from build123d import *

# Parameters (mm, degrees)
F0_R     = 29
F1_DEPTH = 135
F4_DEPTH = 10
F5_DEPTH = 10


with BuildPart() as f1:
    # F0 (on Right) → F1 (new body)
    with BuildSketch(Plane.YZ):
        Circle(F0_R)
    extrude(amount=-F1_DEPTH)

    # F2 (on Right) → F3 (revolve)
    with BuildSketch(Plane.YZ):
        with BuildLine():
            ThreePointArc((0, 16), (3.1819805153, 17.3180194847), (4.5, 20.5))
            ThreePointArc((4.5, 20.5), (-3.1819805153, 23.6819805153), (0, 16))
        make_face()
    revolve(axis=Axis((0, -100, 0), (0, -1, 0)))

    # F4 (add): a face of the model
    f4_faces = [f1.faces().sort_by_distance(p)[0] for p in [
        (-135, 0, 0),
    ]]
    extrude(f4_faces, amount=F4_DEPTH)

    # F5 (cut): a face of the model
    f5_faces = [f1.faces().sort_by_distance(p)[0] for p in [
        (0, 0, 0),
    ]]
    extrude(f5_faces, amount=-F5_DEPTH, mode=Mode.SUBTRACT)


solid = f1.part
Check sheet for the modelled part. Datum: model origin and axes. Units: mm. Round coordinates to 2 decimals unless told otherwise and drop trailing zeros. Loops run counter-clockwise (first coordinate to the right, second up) from the corner with the lowest first, then second, coordinate; pieces in that order, holes last. Notation, with made-up numbers: (-32.75, 67) - (26.25, 67) arc R19 ccw to (26.25, 91) - close; hole circle Ø5 at (19.5, 70.5). An arc over 180 degrees is marked (long way). Answer as CSV lines item,"result". Start each with the question number.
Item 1: Section check A-A (x = -6). Record the boundary of the cut face in (y, z), and give its area (3 significant figures).
Item 2: Section check C-C (x = -45.5). Record the boundary of the cut face in (y, z).
Item 3: Section check D-D (y = 18). Record the boundary of the cut face in (x, z).
Item 4: Depth check by flat-ended pin: P1, Ø6, axis at x = -72.5, y = 18.5, coming from the +Z side; P2, Ø12, axis at x = -107, y = 6.5, coming from the +Z side; P3, Ø4, axis at y = 0, z = -9.5, coming from the +X side. Enter the tip coordinate at first touch or a pass-through.
Item 5: Section check B-B (y = -16.5). Record the boundary of the cut face in (x, z).
Item 6: Scan lines: line 1 (X direction, y = 25, z = 13.5); line 2 (Y direction, x = -36, z = 20.5); line 3 (X direction, y = 3.5, z = 13.5). Record each from-to range of solid material in increasing order. Write a range as [from, to].
Report:
1,outline,"circle Ø9 at (0, -20.5); circle Ø9 at (0, 20.5)"
1,area,"127 mm2"
2,outline,"circle Ø58 at (0, 0)"
3,outline,"(-145, -22.74) - (-10, -22.74) - (-10, 22.74) - (-145, 22.74) - close"
4,P1,"stops at z = 24.51"
4,P2,"stops at z = 29"
4,P3,"stops at x = 23.85"
5,outline,"(-145, -23.85) - (-10, -23.85) - (-10, 23.85) - (-145, 23.85) - close"
6,line 1,"x = [-145, -10]"
6,line 2,"y = [-20.51, 20.51]"
6,line 3,"x = [-145, -10], [11.4, 19.03]"
